Work out the finished part from the listing and answer in its coordinate system (mm). A direction names the side the tool comes from. Round coordinates to 2 decimals unless told otherwise and drop trailing zeros. Loops run counter-clockwise (first coordinate to the right, second up) from the corner with the lowest first, then second, coordinate; pieces in that order, holes last. Notation, with made-up numbers: (48, 53) - (59, 53) arc R21 ccw to (59, 68) - close; hole circle Ø5 at (83, 45). An arc over 180 degrees is marked (long way). Return JSON: item names as keys, results as strings.
from build123d import *

# Parameters (mm, degrees)
SKETCH1_W           = 44
SKETCH1_H           = 48
BOSS_EXTRUDE1_DEPTH = 7
SKETCH2_W           = 42.2
SKETCH2_H           = 46
CUT_EXTRUDE1_DEPTH  = 6.5
CUT_EXTRUDE2_REACH  = 67.439
SKETCH3_W           = 31
SKETCH3_H           = 37
SKETCH4_W           = 8
SKETCH4_H           = 46
BOSS_EXTRUDE2_DEPTH = 2
SKETCH5_W           = 0.8
SKETCH5_H           = 24
CUT_EXTRUDE3_DEPTH  = 3
FILLET1_R           = 2
FILLET2_R           = 1
SKETCH6_W           = 3
SKETCH6_H           = 20
CUT_EXTRUDE4_DEPTH  = 1.5


with BuildPart() as part:
    # Sketch1 → Boss-Extrude1 (new body)
    with BuildSketch(Plane(origin=(0, 0, 0), x_dir=(1, 0, 0), z_dir=(0, 1, 0))):
        with Locations((22, 24)):
            Rectangle(SKETCH1_W, SKETCH1_H)
    extrude(amount=BOSS_EXTRUDE1_DEPTH)

    # Sketch2 → Cut-Extrude1 (cut)
    with BuildSketch(Plane(origin=(0, 7, 0), x_dir=(1, 0, 0), z_dir=(0, 1, 0))):
        with Locations((22.1, 24)):
            Rectangle(SKETCH2_W, SKETCH2_H)
    extrude(amount=-CUT_EXTRUDE1_DEPTH, mode=Mode.SUBTRACT)

    # Sketch3 → Cut-Extrude2 (cut, up to next)
    with BuildSketch(Plane(origin=(0, 0.5, 0), x_dir=(1, 0, 0), z_dir=(0, 1, 0)), mode=Mode.PRIVATE) as cut_extrude2_sk1:
        with Locations((18, 27)):
            Rectangle(SKETCH3_W, SKETCH3_H)
    cut_extrude2_tool1 = extrude(cut_extrude2_sk1.sketch, amount=-CUT_EXTRUDE2_REACH, mode=Mode.PRIVATE) & part.part
    add(cut_extrude2_tool1.solids().sort_by_distance((18, 0.5, -27))[0], mode=Mode.SUBTRACT)

    # Sketch4 → Boss-Extrude2 (add)
    with BuildSketch(Plane(origin=(0, 0.5, 0), x_dir=(1, 0, 0), z_dir=(0, 1, 0))):
        with Locations((39.2, 24)):
            Rectangle(SKETCH4_W, SKETCH4_H)
    extrude(amount=BOSS_EXTRUDE2_DEPTH)

    # Sketch5 → Cut-Extrude3 (cut)
    with BuildSketch(Plane(origin=(0, 7, 0), x_dir=(1, 0, 0), z_dir=(0, 1, 0))):
        with Locations((43.6, 33)):
            Rectangle(SKETCH5_W, SKETCH5_H)
    extrude(amount=-CUT_EXTRUDE3_DEPTH, mode=Mode.SUBTRACT)

    # Fillet1
    fillet1_edges = [part.edges().sort_by_distance(p)[0] for p in [
        (0, 3.5, -48),
        (0, 3.5, 0),
    ]]
    fillet(fillet1_edges, radius=FILLET1_R)

    # Fillet2
    fillet2_edges = [part.edges().sort_by_distance(p)[0] for p in [
        (2.5, 0.25, -8.5),
        (2.5, 0.25, -45.5),
        (33.5, 0.25, -45.5),
        (33.5, 0.25, -8.5),
    ]]
    fillet(fillet2_edges, radius=FILLET2_R)

    # Sketch6 → Cut-Extrude4 (cut)
    with BuildSketch(Plane(origin=(0, 2.5, 0), x_dir=(1, 0, 0), z_dir=(0, 1, 0))):
        with Locations((38.7, 34)):
            Rectangle(SKETCH6_W, SKETCH6_H)
    extrude(amount=-CUT_EXTRUDE4_DEPTH, mode=Mode.SUBTRACT)


solid = part.part
1) Section A-A (x = 6.5) is taken. Give the vertices of the cut face in (y, z), and give its area (3 significant figures).
Verdict:
{"outline": "(0, -48) - (7, -48) - (7, -47) - (0.5, -47) - (0.5, -45.5) - (0, -45.5) - close; (0, -8.5) - (0.5, -8.5) - (0.5, -1) - (7, -1) - (7, 0) - (0, 0) - close", "area": "18.5 mm2"}
2) Determine the mould class of faces 4 (the flat face through (36, 0, -24)), 5 (the cylindrical face through (33.215, 0.246, -45.199)), 6 (the flat face through (0, 3, -24)), 7 (the flat face through (22, 4, -1)) for opening direction X: pulls with the +X half, pulls with the -X half, needs draft (parallel to the pull), parting line crosses it, or undercut.
Verdict:
{"face 4": "needs draft", "face 5": "undercut", "face 6": "pulls with the -X half", "face 7": "undercut"}
3) Section C-C (y = 5.5) is taken. Give the vertices of the cut face in (x, z), and give its area (3 significant figures).
Verdict:
{"outline": "(0, -46) arc R2 ccw to (2, -48) - (44, -48) - (44, -45) - (43.2, -45) - (43.2, -47) - (1, -47) - (1, -1) - (43.2, -1) - (43.2, -21) - (44, -21) - (44, 0) - (2, 0) arc R2 ccw to (0, -2) - close", "area": "150 mm2"}
4) Find the intervals of material crossed by L1, parallel to X at y = 2, z = -30; L2, parallel to X at y = 6.5, z = -13; L3, parallel to Z at x = 32.5, y = 6.75, in increasing order.
Verdict:
{"L1": "x = 0 to 1, 35.2 to 37.2, 40.2 to 44", "L2": "x = 0 to 1, 43.2 to 44", "L3": "z = -48 to -47, -1 to 0"}
5) A tool of negligible diameter and unlimited length cuts with its end or side. For faces 1 (the cylindrical face through (0.57, 3.55, -47.4)), 2 (the flat face through (37.2, 2, -34)), 3 (the cylindrical face through (2.785, 0.246, -8.801)), from which of +Z, -Z, +X, -X, +Y, -Y can it reach the whole face along a straight path? Write none if from no direction.
Verdict:
{"face 1": "-Z, -X, +Y, -Y", "face 2": "+Y", "face 3": "+Y, -Y"}
6) Section D-D (x = 39.5) is taken. Give the vertices of the cut face in (y, z), and give its area (3 significant figures).
Verdict:
{"outline": "(0, -48) - (7, -48) - (7, -47) - (2.5, -47) - (2.5, -44) - (1, -44) - (1, -24) - (2.5, -24) - (2.5, -1) - (7, -1) - (7, 0) - (0, 0) - close", "area": "99.0 mm2"}
7) Flat-ended cylindrical pins translate along their axes: pin 1 (1 mm diameter, centred on x = 34, z = -16, fed in from +Y); pin 2 (1.5 mm diameter, centred on x = 38, z = -29, fed in from +Y); pin 3 (4 mm diameter, centred on x = 40, z = -31.5, fed in from +Y). Find the tip coordinate at first contact, or state that the pin passes through.
Verdict:
{"pin 1": "stops at y = 0.5", "pin 2": "stops at y = 1", "pin 3": "stops at y = 2.5"}
8) Section B-B (z = -18) is taken. Give the vertices of the cut face in (x, y), and give its area (3 significant figures).
Verdict:
{"outline": "(0, 0) - (2.5, 0) - (2.5, 0.5) - (1, 0.5) - (1, 7) - (0, 7) - close; (33.5, 0) - (44, 0) - (44, 7) - (43.2, 7) - (43.2, 2.5) - (35.2, 2.5) - (35.2, 0.5) - (33.5, 0.5) - close", "area": "34.2 mm2"}
